from build123d import *

# Parameters (mm, degrees)
EXTRUDE_1_DEPTH                  = 150
SKETCH_10_W                      = 150
SKETCH_10_H                      = 201.944841161
CUT_EXTRUDE_9_DEPTH              = 232.130644437
PATTERN_CIRCULAR_6_COUNT         = 8
EXTRUDE_6_DEPTH                  = 150
CUT_EXTRUDE_10_REACH             = 194.224
CUT_EXTRUDE_10_DIRECTION_2_REACH = 194.224
PATTERN_CIRCULAR_7_COUNT         = 8
EXTRUDE_7_DEPTH                  = 150


with BuildPart() as part:
    # 草图1 → 凸台-拉伸1 (new body)
    with BuildSketch(Plane(origin=(0, 0, 0), x_dir=(1, 0, 0), z_dir=(0, 1, 0))):
        Polygon((-60.104076401, -60.104076401), (0, -85), (60.104076401, -60.104076401), (85, 0), (60.104076401, 60.104076401), (0, 85), (-60.104076401, 60.104076401), (-85, 0), align=None)
        Polygon((-15.307337295, -36.9551813), (15.307337295, -36.9551813), (36.9551813, -15.307337295), (36.9551813, 15.307337295), (15.307337295, 36.9551813), (-15.307337295, 36.9551813), (-36.9551813, 15.307337295), (-36.9551813, -15.307337295), align=None, mode=Mode.SUBTRACT)
    extrude(amount=EXTRUDE_1_DEPTH)

    # 草图10 → 切除-拉伸9 (cut, through all)
    with BuildSketch(Plane(origin=(-28.191943273, 18.923017893, 68.0613718), x_dir=(0.9287722113346277, 0.09928567118319402, 0.35710577557677253), z_dir=(-0.3706510211136421, 0.2487886640689572, 0.894830722079991))):
        with Locations((13.456718785, 57.315220344)):
            Rectangle(SKETCH_10_W, SKETCH_10_H)
    cut_extrude_9 = extrude(amount=CUT_EXTRUDE_9_DEPTH, mode=Mode.SUBTRACT)

    # 阵列(圆周)6: 切除-拉伸9 ×8 about axis
    pattern_circular_6_axis = Axis((0, 0, 0), (0, 1, 0))
    for i in range(1, PATTERN_CIRCULAR_6_COUNT):
        add(cut_extrude_9.rotate(pattern_circular_6_axis, i * 360 / PATTERN_CIRCULAR_6_COUNT), mode=Mode.SUBTRACT)

    # 草图13 → 凸台-拉伸6 (add, through all)
    with BuildSketch(Plane(origin=(0, 0, 0), x_dir=(1, 0, 0), z_dir=(0, 1, 0))):
        Polygon((-36.9551813, 15.307337295), (-85, 0), (-36.9551813, -15.307337295), align=None)
    extrude_6 = extrude(amount=EXTRUDE_6_DEPTH)

    # 草图14 → 切除-拉伸10 (cut, up to next)
    with BuildSketch(Plane.XY, mode=Mode.PRIVATE) as cut_extrude_10_sk1:
        Polygon((-36.9551813, 150), (-85, 150), (-85, 100), align=None)
    cut_extrude_10_tool1 = extrude(cut_extrude_10_sk1.sketch, amount=-CUT_EXTRUDE_10_REACH, mode=Mode.PRIVATE) & part.part
    cut_extrude_10 = cut_extrude_10_tool1.solids().sort_by_distance((-68.98506, 133.333333, 0))[0]
    add(cut_extrude_10, mode=Mode.SUBTRACT)

    # 草图14 → 切除-拉伸10 direction 2 (cut, up to next)
    with BuildSketch(Plane.XY, mode=Mode.PRIVATE) as cut_extrude_10_direction_2_sk1:
        Polygon((-36.9551813, 150), (-85, 150), (-85, 100), align=None)
    cut_extrude_10_direction_2_tool1 = extrude(cut_extrude_10_direction_2_sk1.sketch, amount=CUT_EXTRUDE_10_DIRECTION_2_REACH, mode=Mode.PRIVATE) & part.part
    cut_extrude_10_direction_2 = cut_extrude_10_direction_2_tool1.solids().sort_by_distance((-68.98506, 133.333333, 0))[0]
    add(cut_extrude_10_direction_2, mode=Mode.SUBTRACT)

    # 阵列(圆周)7: 凸台-拉伸6, 切除-拉伸10, 切除-拉伸10 direction 2 ×8 about axis
    pattern_circular_7_axis = Axis((0, 0, 0), (0, 1, 0))
    add([extrude_6.rotate(pattern_circular_7_axis, i * 360 / PATTERN_CIRCULAR_7_COUNT) for i in range(1, PATTERN_CIRCULAR_7_COUNT)])
    add([cut_extrude_10.rotate(pattern_circular_7_axis, i * 360 / PATTERN_CIRCULAR_7_COUNT) for i in range(1, PATTERN_CIRCULAR_7_COUNT)], mode=Mode.SUBTRACT)
    add([cut_extrude_10_direction_2.rotate(pattern_circular_7_axis, i * 360 / PATTERN_CIRCULAR_7_COUNT) for i in range(1, PATTERN_CIRCULAR_7_COUNT)], mode=Mode.SUBTRACT)

    # 草图1<3> → 凸台-拉伸7 (add)
    with BuildSketch(Plane(origin=(0, 0, 0), x_dir=(1, 0, 0), z_dir=(0, 1, 0))):
        Polygon((-36.9551813, -15.307337295), (-15.307337295, -36.9551813), (15.307337295, -36.9551813), (36.9551813, -15.307337295), (36.9551813, 15.307337295), (15.307337295, 36.9551813), (-15.307337295, 36.9551813), (-36.9551813, 15.307337295), align=None)
        Polygon((13.236269483, 31.9551813), (-13.236269483, 31.9551813), (-31.9551813, 13.236269483), (-31.9551813, -13.236269483), (-13.236269483, -31.9551813), (13.236269483, -31.9551813), (31.9551813, -13.236269483), (31.9551813, 13.236269483), align=None, mode=Mode.SUBTRACT)
    extrude(amount=EXTRUDE_7_DEPTH)


solid = part.part
Geometry: final body of the model. Coordinates: model frame, mm. A direction names the side the tool comes from. Coordinates: 2 decimals unless noted, no trailing zeros. Loops run counter-clockwise (first coordinate to the right, second up) from the corner with the lowest first, then second, coordinate; pieces in that order, holes last. Notation, with made-up numbers: (-14.5, 0) - (30.5, 0) arc R12 cw to (30.5, 19) - close; hole circle Ø1 at (-1, 77.5). An arc over 180 degrees is marked (long way). Put each result on its own line as item: value. Start each with the question number.
Q1. Pin query (flat end, axial travel): pin 1 Ø3 at (x, y) = (19, 52.5) entering from -Z; pin 2 Ø8 at (x, z) = (-23, 18) entering from +Y; pin 3 Ø13 at (x, y) = (6, 80) entering from -Z; pin 4 Ø2 at (y, z) = (39, 11) entering from -X. Return the tip coordinate at first contact, or that it passes through.
Q2. Pull-direction query (Z, two-part tool) for faces 1 (the flat face through (-55.976, 130.206, 0.214)), 2 (the flat face through (-22.46, 73.95, -22.73)), 3 (the flat face through (0, 74, 31.955)), 4 (the flat face through (-39.429, 130.206, 39.732)); classes: released by +Z, released by -Z, zero draft, split by the parting line, or undercut.
Q3. Cut plane D-D, the plane x = -51.5. Return loops of the section in (y, z), and give its area (3 significant figures).
Q4. Line query: line 1 (X direction, y = 33, z = -59); line 2 (X direction, y = 68.5, z = -51); line 3 (Z direction, x = 53, y = 76). Output: solid intervals per line, ascending.
Q5. Cut plane A-A, the plane z = -22.5. Return loops of the section in (x, y).
Q6. Cut plane C-C, the plane x = 3.5. Return loops of the section in (y, z).
Q7. Set-up query: faces 5 (the flat face through (-46.106, 85.761, 52.87)), 6 (the flat face through (-39.732, 130.206, -39.429)), 7 (the flat face through (-31.955, 74, 0)), 8 (the flat face through (52.87, 85.761, 46.106)). Return all of +Z, -Z, +X, -X, +Y, -Y with unobstructed straight access to the full face (end or side cutting, diameter ignored); none if empty.
Filled sheet:
1. pin 1: z = -63.28
1. pin 2: y = 150
1. pin 3: z = -85
1. pin 4: x = -70.1
2. face 1: zero draft
2. face 2: undercut
2. face 3: undercut
2. face 4: released by +Z
3. outline: (0, -63.67) - (28.81, -55.66) - (109.6, -55.66) - (118.58, -43.45) - (55.75, -43.45) - (104.59, -10.67) - (134.86, -10.67) - (134.86, 10.67) - (104.59, 10.67) - (55.75, 43.45) - (118.58, 43.45) - (109.6, 55.66) - (28.81, 55.66) - (0, 63.67) - close
3. area: 11,200 mm²
4. line 1: -59.53 to -57.97, -40.62 to 40.62, 57.97 to 59.53
4. line 2: -55.4 to -42.49, -36.1 to 36.1, 42.49 to 55.4
4. line 3: -56.43 to -46.36, -26.24 to 26.24, 46.36 to 56.43
5. outline: (-75.68, 0) - (-22.69, 0) - (-22.69, 150) - (-29.76, 150) - (-40.67, 141.97) - (-40.67, 125.92) - close; (22.69, 0) - (75.68, 0) - (40.67, 125.92) - (40.67, 141.97) - (29.76, 150) - (22.69, 150) - close
6. outline: (0, -83.55) - (34.3, -74.01) - (111.43, -74.01) - (150, -36.96) - (150, -31.96) - (0, -31.96) - close; (0, 31.96) - (150, 31.96) - (150, 36.96) - (111.43, 74.01) - (34.3, 74.01) - (0, 83.55) - close
7. face 5: +Z, +Y
7. face 6: -Z, -X, +Y
7. face 7: +Y, -Y
7. face 8: +X, +Y
